```python
from build123d import *

# Parameters (mm, degrees)
F0_R     = 77.066086
F1_DEPTH = 25.4
F3_DEPTH = 25.4


with BuildPart() as f1:
    # F0 (on Right) → F1 (new body)
    with BuildSketch(Plane.YZ):
        Circle(F0_R)
    extrude(amount=F1_DEPTH)

    # F2 (on face) → F3 (cut)
    with BuildSketch(Plane(origin=(0, 0, 0), x_dir=(0, -1, 0), z_dir=(-1, 0, 0))):
        Polygon((51.66469, 13.667783), (13.995698, 51.576825), (-37.668992, 37.909042), (-51.66469, -13.667783), (-13.995698, -51.576825), (37.668992, -37.909042), align=None)
    extrude(amount=-F3_DEPTH, mode=Mode.SUBTRACT)


solid = f1.part
```
Check sheet for the modelled part. Datum: model origin and axes. Units: mm. A direction names the side the tool comes from. Coordinates: 2 decimals unless noted, no trailing zeros. Loops run counter-clockwise (first coordinate to the right, second up) from the corner with the lowest first, then second, coordinate; pieces in that order, holes last.
1) Access from +Z, -Z, +X, -X, +Y, -Y to the whole of each face (thin tool, end or side, straight path). Record for faces 1 (the face through (12.52, -44.57, -12.48)), 2 (the face through (0, 33, -33)).
2) Sectioned sample at D-D (y = 59). Record the boundary of the cut face in (x, z), and give its area (3 significant figures).
3) Sectioned sample at A-A (y = -2). Record the boundary of the cut face in (x, z).
4) Gauge pin test, flat ends, axial feed: pin 1 (6 mm diameter, centred on x = 23, y = -30, fed in from -Z); pin 2 (10 mm diameter, centred on x = 17.5, z = 13.5, fed in from -Y); pin 3 (10 mm diameter, centred on x = 7.5, z = 11.5, fed in from +Y). Record the tip position at first contact, or that the pin passes through.
5) Material ranges on probe 1 along Y at (x, z) = (10.75, 34.5); probe 2 along Z at (x, y) = (16.25, -7); probe 3 along Y at (x, z) = (22, 33), recorded low to high.
6) Release check for a two-part mould opening along Y. For faces 3 (the face through (12.52, 71.19, -29.52)), 4 (the face through (12.52, 11.47, 44.84)), 5 (the face through (25.4, 33, -33)) record: released by +Y, released by -Y, zero draft, split by the parting line, or undercut.
7) Sectioned sample at B-B (z = 0). Record the boundary of the cut face in (x, y), and give its area (3 significant figures).
8) Sectioned sample at C-C (x = 19.75). Record the boundary of the cut face in (y, z).
Check sheet entries:
1. face 1: +X, -X
1. face 2: +Z, -Z, -X, +Y, -Y
2. outline: (0, -49.58) - (25.4, -49.58) - (25.4, 49.58) - (0, 49.58) - close
2. area: 2,520 mm2
3. outline: (0, -77.04) - (25.4, -77.04) - (25.4, -47.35) - (0, -47.35) - close; (0, 48.4) - (25.4, 48.4) - (25.4, 77.04) - (0, 77.04) - close
4. pin 1: stops at z = -72.18
4. pin 2: stops at y = -76.6
4. pin 3: stops at y = 76.79
5. probe 1: y = -68.91 to -30.96, 38.59 to 68.91
5. probe 2: z = -76.75 to -46.02, 49.73 to 76.75
5. probe 3: y = -69.64 to -32.45, 39 to 69.64
6. face 3: split by the parting line
6. face 4: undercut
6. face 5: zero draft
7. outline: (0, -77.07) - (25.4, -77.07) - (25.4, -47.96) - (0, -47.96) - close; (0, 47.96) - (25.4, 47.96) - (25.4, 77.07) - (0, 77.07) - close
7. area: 1,480 mm2
8. outline: circle Ø154.13 at (0, 0); hole (-51.66, 13.67) - (-37.67, -37.91) - (14, -51.58) - (51.66, -13.67) - (37.67, 37.91) - (-14, 51.58) - close
